Verification items for the finished model (mm, model axes). A direction names the side the tool comes from. Coordinates: 2 decimals unless noted, no trailing zeros. Loops run counter-clockwise (first coordinate to the right, second up) from the corner with the lowest first, then second, coordinate; pieces in that order, holes last. Notation, with made-up numbers: (-38.5, 13.25) - (8.5, 13.25) arc R11 cw to (8.5, 17.25) - close; hole circle Ø1 at (6, 65). An arc over 180 degrees is marked (long way). Answer as CSV lines item,"result". Start each with the question number.
1. Cross-section at D-D (y = 10). Enter the section's corners in (x, z), plus the area to 3 significant figures.
2. Release check for a two-part mould opening along Z. For faces 3 (the flat face through (0, 0, 0)), 4 (the cylindrical face through (11.446, 42.532, -3.604)), 5 (the cylindrical face through (-0.17, 7.56, 0.54)) record: pulls with the +Z half, pulls with the -Z half, needs draft (parallel to the pull), parting line crosses it, or undercut.
3. Cross-section at B-B (x = 0). Enter the section's corners in (y, z), plus the area to 3 significant figures.
4. Cross-section at C-C (y = 29.5). Enter the section's corners in (x, z), plus the area to 3 significant figures.
5. Set-up check for faces 1 (the flat face through (0, 92, 0)), 2 (the flat face through (0.3, 80, 12.4)): record each of +Z, -Z, +X, -X, +Y, -Y from which the full face is reachable in a straight line by a thin tool's end or side.
6. Gauge pin test, flat ends, axial feed: P1, Ø5, axis at y = 67, z = 8.5, coming from the -X side; P2, Ø3, axis at x = 8.5, y = 33, coming from the +Z side; P3, Ø10, axis at x = 11, y = 23.5, coming from the +Z side. Record the tip position at first contact, or that the pin passes through.
7. Material ranges on line 1 (Y direction, x = 1, z = 0); line 2 (Y direction, x = 13.5, z = 2); line 3 (Z direction, x = -5, y = 10), recorded low to high. Write a range as [from, to].
8. Cross-section at A-A (z = 0). Enter the section's corners in (x, y).
```python
from build123d import *

# Parameters (mm, degrees)
CUT_EXTRUDE1_DEPTH      = 96.843622656
CUT_EXTRUDE1_DEPTH_BACK = 96.843622656
SKETCH2_R               = 2.5


with BuildPart() as part:
    # Sketch1 → Revolve1 (revolve)
    with BuildSketch(Plane.XY):
        with BuildLine():
            Line((0, 0), (8, 0))
            ThreePointArc((8, 0), (10.828427125, 1.171572875), (12, 4))
            Line((12, 4), (12, 80))
            Line((12, 80), (19, 80))
            Line((19, 80), (19, 88))
            ThreePointArc((19, 88), (17.828427125, 90.828427125), (15, 92))
            Line((15, 92), (0, 92))
            Line((0, 92), (0, 0))
        make_face()
    revolve(axis=Axis((0, -790.652262501, 0), (0, 1, 0)))

    # Sketch2 → Cut-Extrude1 (cut, two sides: drawn at the far end of the back side and taken through both)
    with BuildSketch(Plane(origin=(0, 0, 0), x_dir=(0, 0, -1), z_dir=(1, 0, 0)).offset(-CUT_EXTRUDE1_DEPTH_BACK)):
        with Locations((0, 10)):
            Circle(SKETCH2_R)
    extrude(amount=CUT_EXTRUDE1_DEPTH + CUT_EXTRUDE1_DEPTH_BACK, mode=Mode.SUBTRACT)


solid = part.part
```
Values follow:
1,outline,"(-11.74, -2.5) arc R12 ccw to (11.74, -2.5) - close; (-11.74, 2.5) - (11.74, 2.5) arc R12 ccw to start"
1,area,"333 mm²"
2,face 3,"needs draft"
2,face 4,"parting line crosses it"
2,face 5,"undercut"
3,outline,"(0, -8) arc R4 ccw to (4, -12) - (80, -12) - (80, -19) - (88, -19) arc R4 ccw to (92, -15) - (92, 15) arc R4 ccw to (88, 19) - (80, 19) - (80, 12) - (4, 12) arc R4 ccw to (0, 8) - close; hole circle Ø5 at (10, 0)"
3,area,"2,340 mm²"
4,outline,"circle Ø24 at (0, 0)"
4,area,"452 mm²"
5,face 1,"+Z, -Z, +X, -X, +Y"
5,face 2,"-Y"
6,P1,"stops at x = -10.39"
6,P2,"stops at z = 9.75"
6,P3,"stops at z = 10.39"
7,line 1,"y = [0, 7.5], [12.5, 92]"
7,line 2,"y = [80, 92]"
7,line 3,"z = [-10.91, -2.5], [2.5, 10.91]"
8,outline,"(-19, 80) - (-12, 80) - (-12, 12.5) - (12, 12.5) - (12, 80) - (19, 80) - (19, 88) arc R4 ccw to (15, 92) - (-15, 92) arc R4 ccw to (-19, 88) - close; (-12, 4) arc R4 ccw to (-8, 0) - (8, 0) arc R4 ccw to (12, 4) - (12, 7.5) - (-12, 7.5) - close"
